Autodesk Inventor part; units mm, degrees
ref_plane "YZ Plane" through (0, 0, 0) normal (1, 0, 0) x (0, 1, 0)
ref_plane "XZ Plane" through (0, 0, 0) normal (0, 1, 0) x (-1, 0, 0)
ref_plane "XY Plane" through (0, 0, 0) normal (0, 0, 1) x (1, 0, 0)
sketch "Esquisse1" plane through (0, 0, 0) normal (0, 1, 0) x (-1, 0, 0)
  circle A0 centre (8, 0) radius 1
  circle A1 centre (0, 8) radius 1
  circle A2 centre (-8, 0) radius 1
  circle A3 centre (0, -8) radius 1
  line L0 (0, 0) -> (-8, 0) construction
  circle A4 centre (0, 0) radius 11 construction
  line L1 (0, 0) -> (77, 0) construction
  line L2 (0, 0) -> (0, 2.5) construction
  line L3 (0, 2.5) -> (0, 7.5) construction
  line L4 (0, 7.5) -> (8.0467, 7.5) construction
  line L5 (0, 2.5) -> (10.7121, 2.5) construction
  line L6 (11, 0) -> (46, 0) construction
  line L7 (46, 0) -> (51, 0) construction
  line L8 (8.0467, 7.5) -> (51, 7.5)
  line L9 (51, 7.5) -> (51, 0)
  line L10 (10.7121, 2.5) -> (46, 2.5) construction
  line L11 (46, 2.5) -> (46, 0) construction
  line L12 (11, 0) -> (11, 2.5) construction
  arc A5 (8.0467, 7.5) -> (-11, 0) centre (0, 0) ccw
  line L13 (11, 0) -> (13.5, 0) construction
  line L14 (46, 0) -> (43.5, 0) construction
  arc A6 (13.5, 2.5) -> (11, 0) centre (13.5, 0) ccw
  arc A7 (46, 0) -> (43.5, 2.5) centre (43.5, 0) ccw
  line L15 (13.5, 2.5) -> (43.5, 2.5)
  line L16 (8.0467, -7.5) -> (51, -7.5)
  line L17 (51, -7.5) -> (51, 0)
  arc A8 (-11, 0) -> (8.0467, -7.5) centre (0, 0) ccw
  arc A9 (11, 0) -> (13.5, -2.5) centre (13.5, 0) ccw
  arc A10 (43.5, -2.5) -> (46, 0) centre (43.5, 0) ccw
  line L18 (13.5, -2.5) -> (43.5, -2.5)
  circle A11 centre (0, 0) radius 5
  dimension "d7" = 360
  dimension "d12" = 2
  dimension "d13" = 8
  dimension "d14" = 22
  dimension "d19" = 2.5
  dimension "d20" = 5
  dimension "d21" = 35
  dimension "d22" = 5
  dimension "d29" = 10
extrude "Extrusion2" add sketch "Esquisse1" along normal blind 4
fillet "Congé5" radius 5 1 edges at (-51, 2, 7.5)
fillet "Congé6" radius 5 1 edges at (-51, 2, -7.5)
fillet "Congé7" radius 5 1 edges at (-8.0467, 2, 7.5)
fillet "Congé8" radius 5 1 edges at (-8.0467, 2, -7.5)
properties part number "moving_arm"
The model under review builds one solid part; all positions refer to its coordinate system, in mm. A direction names the side the tool comes from. Round coordinates to 2 decimals unless told otherwise and drop trailing zeros. Write each loop counter-clockwise with the first axis right and the second up, starting at its lowest first coordinate (ties: lowest second). Pieces come first, ordered by that corner, then holes. Notation, with made-up numbers: (52.25, -17) -> (104.25, -17) arc R18 cw to (104.25, 14) -> close; hole circle Ø8 at (29.5, 22). An arc over 180 degrees is marked (long way). Use CSV: the item, a comma, the result in double quotes.
Q1. For faces 5 (the flat face through (-28, 2, -2.5)), 6 (the cylindrical face through (4.612, 1.972, -9.987)), list the 3-axis set-ups (+Z, -Z, +X, -X, +Y, -Y) from which the entire face can be reached by the end or side of a thin tool; tool diameter is ignored.
Checks:
face 5,"+Y, -Y"
face 6,"-Z, +Y, -Y"
Q2. To check wall thickness, follow probe 1 along Z at (x, y) = (0, 2.9); probe 2 along Z at (x, y) = (-32, 3.15); probe 3 along Z at (x, y) = (-11.5, 0.7). State the ranges of each line that lie inside material, in increasing order. Write a range as [from, to].
Checks:
probe 1,"[-11, -9], [-7, -5], [5, 7], [9, 11]"
probe 2,"[-7.5, -2.5], [2.5, 7.5]"
probe 3,"[-7.5, -1.5], [1.5, 7.5]"
Q3. Consider section C-C (z = -1.75). Give the boundary of the cut face in (x, y), then the cut area to 3 significant figures.
Checks:
outline,"(-51, 0) -> (-45.29, 0) -> (-45.29, 4) -> (-51, 4) -> close; (-11.71, 0) -> (-4.68, 0) -> (-4.68, 4) -> (-11.71, 4) -> close; (4.68, 0) -> (10.86, 0) -> (10.86, 4) -> (4.68, 4) -> close"
area,"75.7 mm²"
Q4. Mouldability with a two-part tool opening along Z and no side actions: class faces 1 (the flat face through (-28, 2, 2.5)), 2 (the cylindrical face through (-49.57, 2.03, 6)), 3 (the flat face through (-28, 2, -7.5)), 4 (the flat face through (-20, 0, 3)) as released by +Z, released by -Z, zero draft, split by the parting line, or undercut.
Checks:
face 1,"undercut"
face 2,"released by +Z"
face 3,"released by -Z"
face 4,"zero draft"
Q5. Consider section B-B (y = 1.5). Give the boundary of the cut face in (x, z), then the cut area to 3 significant figures.
Checks:
outline,"(-51, -2.5) arc R5 ccw to (-46, -7.5) -> (-9.99, -7.5) arc R5 cw to (-6.87, -8.59) arc R11 ccw to (11, 0) arc R11 ccw to (-6.87, 8.59) arc R5 cw to (-9.99, 7.5) -> (-46, 7.5) arc R5 ccw to (-51, 2.5) -> close; hole (-43.5, -2.5) -> (-13.5, -2.5) arc R2.5 ccw to (-13.5, 2.5) -> (-43.5, 2.5) arc R2.5 ccw to start; hole circle Ø2 at (-8, 0); hole circle Ø10 at (0, 0); hole circle Ø2 at (0, -8); hole circle Ø2 at (0, 8); hole circle Ø2 at (8, 0)"
area,"723 mm²"
Q6. For pin 1 Ø1.5 at (x, y) = (-33, 2) entering from -Z; pin 2 Ø1.5 at (x, y) = (-3.5, 1.5) entering from -Z; pin 3 Ø1.2 at (x, y) = (-28.5, 2) entering from +Z, all flat-tipped, find the tip position at first contact; note any pin that passes through.
Checks:
pin 1,"z = -7.5"
pin 2,"z = -10.65"
pin 3,"z = 7.5"
Q7. Consider section A-A (x = -45). Give the boundary of the cut face in (y, z), then the cut area to 3 significant figures.
Checks:
outline,"(0, -7.5) -> (4, -7.5) -> (4, -2) -> (0, -2) -> close; (0, 2) -> (4, 2) -> (4, 7.5) -> (0, 7.5) -> close"
area,"44.0 mm²"
Q8. Consider section D-D (x = 8). Give the boundary of the cut face in (y, z).
Checks:
outline,"(0, -7.55) -> (4, -7.55) -> (4, -1) -> (0, -1) -> close; (0, 1) -> (4, 1) -> (4, 7.55) -> (0, 7.55) -> close"
